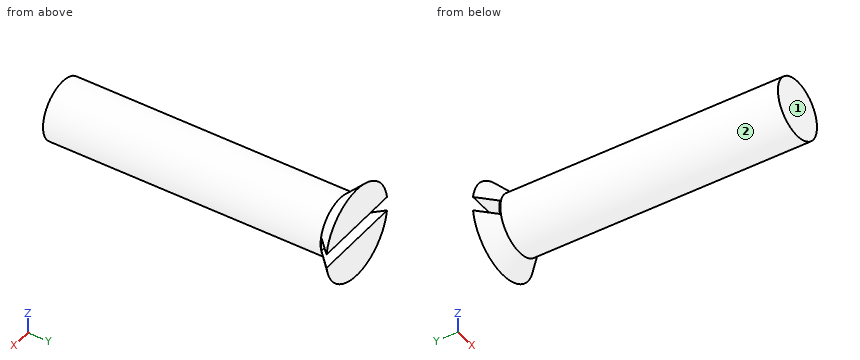
```python
from build123d import *

# Parameters (mm, degrees)
CUT_EXTRUDE1_DEPTH      = 15.320258557
CUT_EXTRUDE1_DEPTH_BACK = 15.320258557
SKETCH2_W               = 1.219880404
SKETCH2_H               = 2.734998975


with BuildPart() as part:
    # Sketch1 → Revolve1 (revolve)
    with BuildSketch(Plane.XY, mode=Mode.PRIVATE) as revolve1_sk:
        Polygon((0, 13.207106781), (-3.914213562, 13.207106781), (-2.5, 11.792893219), (-2.5, -11.792893219), (0, -11.792893219), align=None)
    revolve(revolve1_sk.sketch.rotate(Axis((0, 14.992211838, 0), (0, -1, 0)), 270), axis=Axis((0, 14.992211838, 0), (0, -1, 0)))

    # Sketch2 → Cut-Extrude1 (cut, two sides: drawn at the far end of the back side and taken through both)
    with BuildSketch(Plane(origin=(0, 0, 0), x_dir=(0, 0, -1), z_dir=(1, 0, 0)).offset(-CUT_EXTRUDE1_DEPTH_BACK)):
        with Locations((0, 13.207106782)):
            Rectangle(SKETCH2_W, SKETCH2_H)
    extrude(amount=CUT_EXTRUDE1_DEPTH + CUT_EXTRUDE1_DEPTH_BACK, mode=Mode.SUBTRACT)


solid = part.part
```
Part model, mm, in its own coordinate system. Face numbers are marked on the shaded views. A direction names the side the tool comes from. Round coordinates to 2 decimals unless told otherwise and drop trailing zeros. Order: outer loops, then holes, each group sorted by start corner. A loop starts at its lowest first (then second) coordinate and runs counter-clockwise, first axis right, second up. Notation, with made-up numbers: M -38,62.5 L -22,62.5 A23 cw -22,91.5 Z; hole C 54.25,28 d6. An arc over 180 degrees is marked long. Answer in a Markdown table with one row per item. Add a question column.
Q1. Cut at C-C on y = -7.75. Give the cut face in (x, z), and give its area (3 significant figures).
Q2. Cut at B-B on z = 0. Give the cut face in (x, y), and give its area (3 significant figures).
Q3. 3-axis set-ups, long thin cutter, end or side, ignore diameter. For the marked faces 1 and 2: which of +Z, -Z, +X, -X, +Y, -Y reach the whole face in a straight line?
Q4. Pin check, flat tips, straight feed: pin 1 (3 mm diameter, centred on y = -0.5, z = -0.5, fed in from +X); pin 2 (2 mm diameter, centred on x = -2.5, z = -2.5, fed in from -Y); pin 3 (1 mm diameter, centred on y = -9, z = -2.5, fed in from +X). Stop position of each tip, or through.
Q5. Wall check: L1, parallel to Y at x = -1.25, z = 0.25; L2, parallel to Z at x = 1, y = -10. Give the ranges that are in metal, low to high. Write a range as from..to.
Q6. Cut at A-A on x = 0. Give the cut face in (y, z), and give its area (3 significant figures).
Established:
| question | item | result |
|---|---|---|
| 1 | outline | C 0,0 d5 |
| 1 | area | 19.6 mm2 |
| 2 | outline | M -2.55,11.84 L -2.5,11.79 L -2.5,-11.79 L 2.5,-11.79 L 2.5,11.79 L 2.55,11.84 Z |
| 2 | area | 118 mm2 |
| 3 | face 1 | +Z, -Z, +X, -X, -Y |
| 3 | face 2 | -Y |
| 4 | pin 1 | stops at x = 2.5 |
| 4 | pin 2 | stops at y = 11.83 |
| 4 | pin 3 | stops at x = 1.5 |
| 5 | L1 | y = -11.79..11.84 |
| 5 | L2 | z = -2.29..2.29 |
| 6 | outline | M -11.79,-2.5 L 11.79,-2.5 L 13.21,-3.91 L 13.21,-0.61 L 11.84,-0.61 L 11.84,0.61 L 13.21,0.61 L 13.21,3.91 L 11.79,2.5 L -11.79,2.5 Z |
| 6 | area | 125 mm2 |
